```python
from build123d import *

# Parameters (mm, degrees)
PAD_DEPTH       = 23
POCKET_DEPTH    = 18.001
FILLET_R        = 0.5
SKETCH002_R     = 1.25
POCKET001_DEPTH = 5


with BuildPart() as part:
    # Sketch → Pad (new body)
    with BuildSketch(Plane.XY):
        with BuildLine():
            Line((-9, -13.5), (-9, -3))
            ThreePointArc((-6, 0), (-8.12132, -0.87868), (-9, -3))
            Line((-6, 0), (6, 0))
            ThreePointArc((9, -3), (8.12132, -0.87868), (6, 0))
            Line((9, -3), (9, -13.5))
            Line((9, -13.5), (7.5, -13.5))
            Line((7.5, -13.5), (7.5, -3))
            ThreePointArc((7.5, -3), (7.06066, -1.93934), (6, -1.5))
            Line((6, -1.5), (-6, -1.5))
            ThreePointArc((-6, -1.5), (-7.06066, -1.93934), (-7.5, -3))
            Line((-7.5, -3), (-7.5, -13.5))
            Line((-9, -13.5), (-7.5, -13.5))
        make_face()
    extrude(amount=PAD_DEPTH)

    # Sketch001 (on DatumPlane) → Pocket (cut, through all)
    with BuildSketch(Plane.YZ.offset(9)):
        with BuildLine():
            ThreePointArc((-8.851851, 1.75), (-6, 2.4), (-8.851851, 3.05))
            Line((-8.851851, 3.05), (-14, 3.05))
            Line((-14, 3.05), (-14, 1.75))
            Line((-8.851851, 1.75), (-14, 1.75))
        make_face()
        with BuildLine():
            ThreePointArc((-8.855532, 6.3), (-6.003681, 6.95), (-8.855532, 7.6))
            Line((-8.855532, 7.6), (-14.003681, 7.6))
            Line((-14.003681, 7.6), (-14.003681, 6.3))
            Line((-8.855532, 6.3), (-14.003681, 6.3))
        make_face()
        with BuildLine():
            ThreePointArc((-8.859213, 10.85), (-6.007362, 11.5), (-8.859213, 12.15))
            Line((-8.859213, 12.15), (-14.007362, 12.15))
            Line((-14.007362, 12.15), (-14.007362, 10.85))
            Line((-8.859213, 10.85), (-14.007362, 10.85))
        make_face()
        with BuildLine():
            ThreePointArc((-8.862893, 15.4), (-6.011042, 16.05), (-8.862893, 16.7))
            Line((-8.862893, 16.7), (-14.011042, 16.7))
            Line((-14.011042, 16.7), (-14.011042, 15.4))
            Line((-8.862893, 15.4), (-14.011042, 15.4))
        make_face()
        with BuildLine():
            ThreePointArc((-8.866575, 19.95), (-6.014724, 20.6), (-8.866575, 21.25))
            Line((-8.866575, 21.25), (-14.014724, 21.25))
            Line((-14.014724, 21.25), (-14.014724, 19.95))
            Line((-8.866575, 19.95), (-14.014724, 19.95))
        make_face()
    extrude(amount=-POCKET_DEPTH, mode=Mode.SUBTRACT)

    # Fillet
    fillet_edges = [part.edges().sort_by_distance(p)[0] for p in [
        (-8.25, -13.5, 19.95),
        (-8.25, -13.5, 21.25),
        (-8.25, -13.5, 16.7),
        (-8.25, -13.5, 15.4),
        (-8.25, -13.5, 12.15),
        (-8.25, -13.5, 10.85),
        (-8.25, -13.5, 7.6),
        (-8.25, -13.5, 6.3),
        (-8.25, -13.5, 3.05),
        (-8.25, -13.5, 1.75),
        (8.25, -13.5, 21.25),
        (8.25, -13.5, 19.95),
        (8.25, -13.5, 16.7),
        (8.25, -13.5, 15.4),
        (8.25, -13.5, 12.15),
        (8.25, -13.5, 10.85),
        (8.25, -13.5, 7.6),
        (8.25, -13.5, 6.3),
        (8.25, -13.5, 3.05),
        (8.25, -13.5, 1.75),
    ]]
    fillet(fillet_edges, radius=FILLET_R)

    # Sketch002 (on DatumPlane) → Pocket001 (cut)
    with BuildSketch(Plane(origin=(0, 0, 0), x_dir=(-1, 0, 0), z_dir=(0, 1, 0))):
        with Locations((0, 13)):
            Circle(SKETCH002_R)
    extrude(amount=-POCKET001_DEPTH, mode=Mode.SUBTRACT)


solid = part.part
```
Design review of the part built by this model. Coordinates are the model's own, in mm. A direction names the side the tool comes from. Give positions to 0.01 mm unless a question says otherwise; leave off trailing zeros. Order: outer loops, then holes, each group sorted by start corner. A loop starts at its lowest first (then second) coordinate and runs counter-clockwise, first axis right, second up. Notation, with made-up numbers: (78, 21) -> (109, 21) arc R27 ccw to (109, 39) -> close; hole circle Ø5 at (58, 17). An arc over 180 degrees is marked (long way). Write each question's results on one line, items separated by ' | '. Start each with the question number.
Q1. Mouldability with a two-part tool opening along Z and no side actions: class faces 1 (the flat face through (8, -11, 21.25)), 2 (the cylindrical face through (8.14, -0.9, 11.34)) as +Z half, -Z half, draft (parallel to the pull), parting line (faces both ways), or undercut.
Q2. Wall thickness on L1, parallel to Z at x = 8.05, y = -7.5; L2, parallel to X at y = -3.5, z = 2.75; L3, parallel to X at y = -2, z = 20.5: over which ranges is each line inside the solid? List them lowest first. Write a range as from..to.
Q3. Machinability: for faces 3 (the flat face through (-8, -11, 19.95)), 4 (the flat face through (-7.5, -5.8, 11.3)), 5 (the flat face through (-8, -13.5, 9)), which of the approach directions +Z, -Z, +X, -X, +Y, -Y give a long, thin tool a straight path to every point of the face, cutting with its end or side? Answer none if there is none.
Q4. Add section C-C on z = 20.6. Give the boundary of the cut face in (x, y).
Q5. Add section B-B on y = -5. Give the boundary of the cut face in (x, z).
Q6. Add section A-A on x = 0. Give the boundary of the cut face in (y, z).
Q7. Add section D-D on x = 5.25. Give the boundary of the cut face in (y, z), and give its area (3 significant figures).
Q8. For pin 1 (8 mm diameter, centred on x = 2, y = -1.5, fed in from -Z); pin 2 (2.5 mm diameter, centred on y = -7.5, z = 2.4, fed in from +X), all flat-tipped, find the tip position at first contact; note any pin that passes through.
Found:
1) face 1: undercut | face 2: draft
2) L1: z = 0..0.9, 3.9..5.45, 8.45..10, 13..14.55, 17.55..19.1, 22.1..23 | L2: x = -9..-7.5, 7.5..9 | L3: x = -8.83..-7.12, 7.12..8.83
3) face 3: +X, -X, -Y | face 4: +Z, -Z, -Y | face 5: +Z, -Z, +X, -X, -Y
4) outline: (-9, -6.01) -> (-7.5, -6.01) -> (-7.5, -3) arc R1.5 cw to (-6, -1.5) -> (6, -1.5) arc R1.5 cw to (7.5, -3) -> (7.5, -6.01) -> (9, -6.01) -> (9, -3) arc R3 ccw to (6, 0) -> (-6, 0) arc R3 ccw to (-9, -3) -> close
5) outline: (-9, 0) -> (-7.5, 0) -> (-7.5, 23) -> (-9, 23) -> close; (7.5, 0) -> (9, 0) -> (9, 23) -> (7.5, 23) -> close
6) outline: (-1.5, 0) -> (0, 0) -> (0, 11.75) -> (-1.5, 11.75) -> close; (-1.5, 14.25) -> (0, 14.25) -> (0, 23) -> (-1.5, 23) -> close
7) outline: (-1.5, 0) -> (0, 0) -> (0, 23) -> (-1.5, 23) -> close | area: 34.5 mm2
8) pin 1: stops at z = 0 | pin 2: passes through
